```python
from build123d import *

# Parameters (mm, degrees)
F0_R     = 1
F1_DEPTH = 16
F2_T     = -2.5
F3_DEPTH = 5.3
F4_W     = 11.5
F4_H     = 11.5
F4_R     = 2.75
F4_W_2   = 41.64
F4_H_2   = 10.8
F5_DEPTH = 2.501
F6_SIZE  = 1
F7_SIZE  = 0.5


with BuildPart() as f1:
    # F0 (on Top) → F1 (new body)
    with BuildSketch(Plane.XY):
        with BuildLine():
            Line((26.035, -31.67), (28.575, -31.67))
            ThreePointArc((28.575, -31.67), (33.9065851301, -29.4615851301), (36.115, -24.13))
            Line((36.115, -24.13), (36.115, -21.59))
            Line((36.115, -21.59), (28.575, -21.59))
            ThreePointArc((28.575, -21.59), (26.7789487758, -22.3339487758), (26.035, -24.13))
            Line((26.035, -24.13), (26.035, -31.67))
        make_face()
        with Locations((28.575, -24.13)):
            Circle(F0_R, mode=Mode.SUBTRACT)
        with BuildLine():
            Line((-26.035, -31.67), (26.035, -31.67))
            Line((26.035, -31.67), (26.035, -24.13))
            ThreePointArc((26.035, -24.13), (26.7789487758, -22.3339487758), (28.575, -21.59))
            Line((28.575, -21.59), (36.115, -21.59))
            Line((36.115, -21.59), (36.115, 21.59))
            Line((36.115, 21.59), (28.575, 21.59))
            ThreePointArc((28.575, 21.59), (26.7789487758, 22.3339487758), (26.035, 24.13))
            Line((26.035, 24.13), (26.035, 31.67))
            Line((26.035, 31.67), (-26.035, 31.67))
            Line((-26.035, 31.67), (-26.035, 24.13))
            ThreePointArc((-26.035, 24.13), (-26.7789487758, 22.3339487758), (-28.575, 21.59))
            Line((-28.575, 21.59), (-36.115, 21.59))
            Line((-36.115, 21.59), (-36.115, -21.59))
            Line((-36.115, -21.59), (-28.575, -21.59))
            ThreePointArc((-28.575, -21.59), (-26.7789487758, -22.3339487758), (-26.035, -24.13))
            Line((-26.035, -24.13), (-26.035, -31.67))
        make_face()
        with BuildLine():
            Line((-31.115, -31.67), (-26.035, -31.67))
            Line((-26.035, -31.67), (-26.035, -24.13))
            ThreePointArc((-26.035, -24.13), (-26.7789487758, -22.3339487758), (-28.575, -21.59))
            Line((-28.575, -21.59), (-36.115, -21.59))
            Line((-36.115, -21.59), (-36.115, -26.67))
            ThreePointArc((-36.115, -26.67), (-34.6505339059, -30.2055339059), (-31.115, -31.67))
        make_face()
        with Locations((-31.115, -26.67)):
            Circle(F0_R, mode=Mode.SUBTRACT)
        with BuildLine():
            Line((-36.115, 26.67), (-36.115, 21.59))
            Line((-36.115, 21.59), (-28.575, 21.59))
            ThreePointArc((-28.575, 21.59), (-26.7789487758, 22.3339487758), (-26.035, 24.13))
            Line((-26.035, 24.13), (-26.035, 31.67))
            Line((-26.035, 31.67), (-31.115, 31.67))
            ThreePointArc((-31.115, 31.67), (-34.6505339059, 30.2055339059), (-36.115, 26.67))
        make_face()
        with Locations((-31.115, 26.67)):
            Circle(F0_R, mode=Mode.SUBTRACT)
        with BuildLine():
            Line((28.575, 21.59), (36.115, 21.59))
            Line((36.115, 21.59), (36.115, 26.67))
            ThreePointArc((36.115, 26.67), (34.6505339059, 30.2055339059), (31.115, 31.67))
            Line((31.115, 31.67), (26.035, 31.67))
            Line((26.035, 31.67), (26.035, 24.13))
            ThreePointArc((26.035, 24.13), (26.7789487758, 22.3339487758), (28.575, 21.59))
        make_face()
        with Locations((31.115, 26.67)):
            Circle(F0_R, mode=Mode.SUBTRACT)
        with Locations((31.115, 26.67)):
            Circle(F0_R)
        with Locations((-31.115, 26.67)):
            Circle(F0_R)
        with Locations((-31.115, -26.67)):
            Circle(F0_R)
        with Locations((28.575, -24.13)):
            Circle(F0_R)
    extrude(amount=F1_DEPTH)

    # F2
    f2_openings = [f1.faces().sort_by_distance(p)[0] for p in [
        (-0.051092, 0.04441, 16),
    ]]
    offset(amount=F2_T, openings=f2_openings)

    # F0 (on Top) → F3 (join)
    with BuildSketch(Plane.XY):
        with BuildLine():
            Line((-31.115, -31.67), (-26.035, -31.67))
            Line((-26.035, -31.67), (-26.035, -24.13))
            ThreePointArc((-26.035, -24.13), (-26.7789487758, -22.3339487758), (-28.575, -21.59))
            Line((-28.575, -21.59), (-36.115, -21.59))
            Line((-36.115, -21.59), (-36.115, -26.67))
            ThreePointArc((-36.115, -26.67), (-34.6505339059, -30.2055339059), (-31.115, -31.67))
        make_face()
        with Locations((-31.115, -26.67)):
            Circle(F0_R, mode=Mode.SUBTRACT)
        with BuildLine():
            Line((26.035, -31.67), (28.575, -31.67))
            ThreePointArc((28.575, -31.67), (33.9065851301, -29.4615851301), (36.115, -24.13))
            Line((36.115, -24.13), (36.115, -21.59))
            Line((36.115, -21.59), (28.575, -21.59))
            ThreePointArc((28.575, -21.59), (26.7789487758, -22.3339487758), (26.035, -24.13))
            Line((26.035, -24.13), (26.035, -31.67))
        make_face()
        with Locations((28.575, -24.13)):
            Circle(F0_R, mode=Mode.SUBTRACT)
        with BuildLine():
            Line((28.575, 21.59), (36.115, 21.59))
            Line((36.115, 21.59), (36.115, 26.67))
            ThreePointArc((36.115, 26.67), (34.6505339059, 30.2055339059), (31.115, 31.67))
            Line((31.115, 31.67), (26.035, 31.67))
            Line((26.035, 31.67), (26.035, 24.13))
            ThreePointArc((26.035, 24.13), (26.7789487758, 22.3339487758), (28.575, 21.59))
        make_face()
        with Locations((31.115, 26.67)):
            Circle(F0_R, mode=Mode.SUBTRACT)
        with BuildLine():
            Line((-36.115, 26.67), (-36.115, 21.59))
            Line((-36.115, 21.59), (-28.575, 21.59))
            ThreePointArc((-28.575, 21.59), (-26.7789487758, 22.3339487758), (-26.035, 24.13))
            Line((-26.035, 24.13), (-26.035, 31.67))
            Line((-26.035, 31.67), (-31.115, 31.67))
            ThreePointArc((-31.115, 31.67), (-34.6505339059, 30.2055339059), (-36.115, 26.67))
        make_face()
        with Locations((-31.115, 26.67)):
            Circle(F0_R, mode=Mode.SUBTRACT)
    extrude(amount=F3_DEPTH)

    # F4 (on face) → F5 (cut, through all)
    with BuildSketch(Plane.XY.offset(2.5)):
        with Locations((-18.415, 13.97)):
            Rectangle(F4_W, F4_H)
        with Locations((-18.415, -6.35)):
            Rectangle(F4_W, F4_H)
        with Locations((-5.715, 13.97)):
            Circle(F4_R)
        with Locations((-5.715, -6.35)):
            Circle(F4_R)
        with Locations((6.585, -6.35)):
            Rectangle(F4_W, F4_H)
        with Locations((6.585, 13.97)):
            Rectangle(F4_W, F4_H)
        with Locations((19.285, 13.97)):
            Circle(F4_R)
        with Locations((19.285, -6.35)):
            Circle(F4_R)
        with Locations((0.365, -21.42)):
            Rectangle(F4_W_2, F4_H_2)
    extrude(amount=-F5_DEPTH, mode=Mode.SUBTRACT)

    # F6
    f6_edges = [f1.edges().sort_by_distance(p)[0] for p in [
        (-36.115, 0, 16),
        (-34.650534, 30.205534, 16),
        (0, 31.67, 16),
        (34.650534, 30.205534, 16),
        (36.115, 1.27, 16),
        (33.906585, -29.461585, 16),
        (-1.27, -31.67, 16),
        (-34.650534, -30.205534, 0),
        (-34.650534, -30.205534, 16),
        (33.906585, -29.461585, 0),
        (-1.27, -31.67, 0),
        (36.115, 1.27, 0),
        (-36.115, 0, 0),
        (34.650534, 30.205534, 0),
        (-34.650534, 30.205534, 0),
        (0, 31.67, 0),
    ]]
    chamfer(f6_edges, length=F6_SIZE)

    # F7
    f7_edges = [f1.edges().sort_by_distance(p)[0] for p in [
        (-31.095, -21.59, 5.3),
        (-26.778949, -22.333949, 5.3),
        (-26.035, -26.65, 5.3),
        (-28.575, -29.17, 5.3),
        (-32.882767, -28.437767, 5.3),
        (-33.615, -24.13, 5.3),
        (-32.115, -26.67, 5.3),
        (31.095, -21.59, 2.5),
        (26.778949, -22.333949, 2.5),
        (33.615, 0, 2.5),
        (26.035, -26.65, 2.5),
        (31.095, 21.59, 2.5),
        (0, -29.17, 2.5),
        (26.778949, 22.333949, 2.5),
        (-26.035, -26.65, 2.5),
        (26.035, 26.65, 2.5),
        (-26.778949, -22.333949, 2.5),
        (0, 29.17, 2.5),
        (-31.095, -21.59, 2.5),
        (-26.035, 26.65, 2.5),
        (-33.615, 0, 2.5),
        (-26.778949, 22.333949, 2.5),
        (-31.095, 21.59, 2.5),
        (-24.165, -6.35, 2.5),
        (-18.415, -12.1, 2.5),
        (-12.665, -6.35, 2.5),
        (-18.415, -0.6, 2.5),
        (-8.465, -6.35, 2.5),
        (0.365, -16.02, 2.5),
        (-20.455, -21.42, 2.5),
        (0.365, -26.82, 2.5),
        (21.185, -21.42, 2.5),
        (0.835, -6.35, 2.5),
        (6.585, -12.1, 2.5),
        (12.335, -6.35, 2.5),
        (6.585, -0.6, 2.5),
        (16.535, -6.35, 2.5),
        (-18.415, 8.22, 2.5),
        (-12.665, 13.97, 2.5),
        (-18.415, 19.72, 2.5),
        (-24.165, 13.97, 2.5),
        (-8.465, 13.97, 2.5),
        (6.585, 8.22, 2.5),
        (12.335, 13.97, 2.5),
        (6.585, 19.72, 2.5),
        (0.835, 13.97, 2.5),
        (16.535, 13.97, 2.5),
        (-33.615, 0, 16),
        (-32.115, 26.67, 5.3),
        (0, 29.17, 16),
        (-32.882767, 28.437767, 16),
        (32.882767, 28.437767, 16),
        (30.115, 26.67, 5.3),
        (26.035, -26.65, 5.3),
        (26.778949, -22.333949, 5.3),
        (31.095, -21.59, 5.3),
        (33.615, -22.86, 5.3),
        (32.138818, -27.693818, 5.3),
        (27.305, -29.17, 5.3),
        (27.575, -24.13, 5.3),
        (32.138818, -27.693818, 16),
        (-1.27, -29.17, 16),
        (-32.882767, -28.437767, 16),
        (33.615, 1.27, 16),
        (-26.035, -29.17, 3.9),
        (26.035, -29.17, 3.9),
        (-33.615, -21.59, 3.9),
        (33.615, -21.59, 3.9),
    ]]
    chamfer(f7_edges, length=F7_SIZE)


solid = f1.part
```
For this review, take the finished solid that the model builds, in its own axes (mm). A direction names the side the tool comes from. Round coordinates to 2 decimals unless told otherwise and drop trailing zeros. Write each loop counter-clockwise with the first axis right and the second up, starting at its lowest first coordinate (ties: lowest second). Pieces come first, ordered by that corner, then holes. Notation, with made-up numbers: (-2, -38) - (15, -38) arc R25 ccw to (15, -25) - close; hole circle Ø3 at (83.5, 44.25). An arc over 180 degrees is marked (long way). Put each result on its own line as item: value.
Q1. Machinability: for faces 1 (the face through (-2, -31.67, 8)), 2 (the face through (29, -24, 2.5)), 3 (the face through (21.185, -21, 1)), which of the approach directions +Z, -Z, +X, -X, +Y, -Y give a long, thin tool a straight path to every point of the face, cutting with its end or side? Answer none if there is none.
Solved:
face 1: +Z, -Z, +X, -X, -Y
face 2: +Z
face 3: +Z, -Z
Q2. We need section B-B (y = -6.35). Count the separate pieces of the cut face and the enclosed holes in it, and give its area (3 significant figures).
Solved:
separate pieces: 5
enclosed holes: 0
area: 160 mm2
Q3. Wall thickness on probe 1 along Y at (x, z) = (12, 1.75); probe 2 along X at (y, z) = (26.67, 3.4) (3 decimals); probe 3 along X at (y, z) = (-4.5, 14.75) (3 decimals): over which ranges is each line inside the solid? List them lowest first.
Solved:
probe 1: y = -31.67 to -26.82, -16.02 to -12.1, -0.6 to 8.22, 19.72 to 31.67
probe 2: x = -36.115 to -32.115, -30.115 to -26.035, 26.035 to 30.115, 32.115 to 36.115
probe 3: x = -36.115 to -33.615, 33.615 to 36.115
Q4. Insertion check: pin 1 Ø1.2 at (x, y) = (28.575, -24.13) entering from +Z; pin 2 Ø3.5 at (x, y) = (-28.5, -25.5) entering from +Z; pin 3 Ø1 at (x, y) = (29, -24.5) entering from +Z. Each pin has a flat end and moves straight along its axis. Give the tip position at first contact, or say it passes through.
Solved:
pin 1: stops at z = 2.5
pin 2: stops at z = 5.3
pin 3: stops at z = 4.86
Q5. We need section A-A (z = 7.5). Give the boundary of the cut face in (x, y) (3 decimals).
Solved:
outline: (-36.115, -26.67) arc R5 ccw to (-31.115, -31.67) - (28.575, -31.67) arc R7.54 ccw to (36.115, -24.13) - (36.115, 26.67) arc R5 ccw to (31.115, 31.67) - (-31.115, 31.67) arc R5 ccw to (-36.115, 26.67) - close; hole (-33.615, -26.67) arc R2.5 ccw to (-31.115, -29.17) - (28.575, -29.17) arc R5.04 ccw to (33.615, -24.13) - (33.615, 26.67) arc R2.5 ccw to (31.115, 29.17) - (-31.115, 29.17) arc R2.5 ccw to (-33.615, 26.67) - close
